CAD build for the part. Positions are in the model's coordinates, mm. Face numbers are marked on the shaded views. A direction names the side the tool comes from. Give positions to 0.01 mm unless a question says otherwise; leave off trailing zeros. Order: outer loops, then holes, each group sorted by start corner. A loop starts at its lowest first (then second) coordinate and runs counter-clockwise, first axis right, second up. Notation, with made-up numbers: M 83.5,34 L 133.5,34 A18 cw 133.5,61 Z; hole C 83.25,5 d5. An arc over 180 degrees is marked long. Put each result on its own line as item: value. Start each with the question number.
1) Cut at B-B (x = -103). Write the cut outline in (y, z).
2) Drill centre lines: line 1 (Z direction, x = -140, y = 17); line 2 (Y direction, x = -92.5, z = 20); line 3 (Y direction, x = -94, z = 9). Where is each one in solid material? Low to high. Write a range as [from, to].
3) Cut at A-A (y = 84). Write the cut outline in (x, z), and give its area (3 significant figures).
4) Pin check, flat tips, straight feed: pin 1 (7.5 mm diameter, centred on y = 74, z = -23.5, fed in from +X); pin 2 (15 mm diameter, centred on x = -15.5, z = -4.5, fed in from -Y); pin 3 (6 mm diameter, centred on x = -125, z = 15.5, fed in from +Y). Stop position of each tip, or through.
5) Tool access for the marked faces 1, 2 and 3: list every direction of +Z, -Z, +X, -X, +Y, -Y with a clear straight run to the whole face (end or side of a thin tool).
6) Cut at C-C (y = 54). Write the cut outline in (x, z), and give its area (3 significant figures).
7) Cut at D-D (y = 110). Write the cut outline in (x, z).
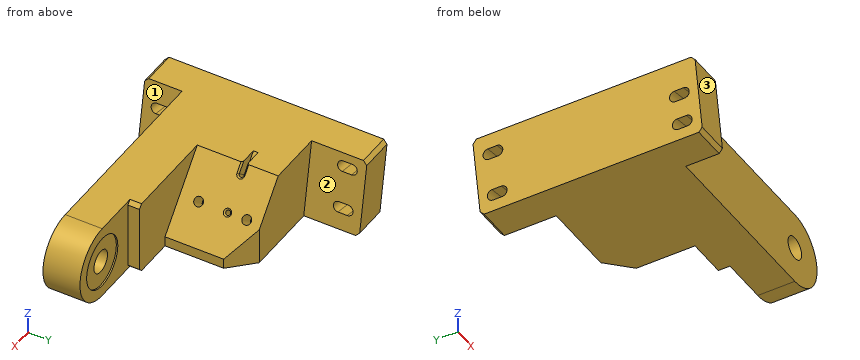
```python
from build123d import *

# Parameters (mm, degrees)
SKETCH1_W                              = 181.864
SKETCH1_H                              = 50.8
EXTRUDE1_DEPTH                         = 152.4
EXTRUDE2_DEPTH                         = 153.4
EXTRUDE3_DEPTH                         = 38.1
EXTRUDE4_DEPTH                         = 55.5498
SKETCH5_W                              = 54.61
SKETCH5_H                              = 50.8
EXTRUDE5_DEPTH                         = 7.9502
EXTRUDE6_DEPTH                         = 25.4
EXTRUDE7_DEPTH                         = 32.584173829
LPATTERN1_COUNT                        = 2
LPATTERN1_PITCH                        = 127
LPATTERN1_COUNT_DIR2                   = 2
LPATTERN1_PITCH_DIR2                   = 27.94
F_1_4_20_TAPPED_HOLE1_D                = 5.1054
F_1_4_20_TAPPED_HOLE1_DEPTH            = 16.51
F_1_4_20_TAPPED_HOLE1_CBORE_D          = 6.35
F_1_4_20_TAPPED_HOLE1_CBORE_DEPTH      = 12.7
F_1_4_20_TAPPED_HOLE1_TIP              = 1.533816902
EXTRUDE9_DEPTH                         = 128
CHAMFER1_SIZE                          = 2.54
CHAMFER2_SIZE                          = 15.24
EXTRUDE10_DEPTH                        = 32.584173829
SCREW_THRU_HOLE_AND_CBORE_D            = 15.4686
SCREW_THRU_HOLE_AND_CBORE_CBORE_D      = 35.56
SCREW_THRU_HOLE_AND_CBORE_CBORE_DEPTH  = 1.016
F_1_8_0_125_DIAMETER_HOLE1_D           = 3.19024
F_1_8_0_125_DIAMETER_HOLE1_DEPTH       = 9.525
F_1_8_0_125_DIAMETER_HOLE1_CSINK_D     = 5.334
F_1_8_0_125_DIAMETER_HOLE1_CSINK_ANGLE = 90
F_1_8_0_125_DIAMETER_HOLE1_TIP         = 0.958444791
CUT_EXTRUDE1_DEPTH                     = 9.525
CHAMFER3_SIZE                          = 1.0795


with BuildPart() as part:
    # Sketch1 → Extrude1 (new body)
    with BuildSketch(Plane(origin=(0, 0, 0), x_dir=(1, 0, 0), z_dir=(0, 1, 0))):
        with Locations((-65.532, 0)):
            Rectangle(SKETCH1_W, SKETCH1_H)
    extrude(amount=EXTRUDE1_DEPTH)

    # Sketch2 → Extrude2 (cut, through all)
    with BuildSketch(Plane(origin=(0, 152.4, 0), x_dir=(1, 0, 0), z_dir=(0, 1, 0))):
        Polygon((-156.464, -25.4), (-156.464, 25.4), (-147.50658938, 25.4), align=None)
    extrude(amount=-EXTRUDE2_DEPTH, mode=Mode.SUBTRACT)

    # Sketch3 → Extrude3 (cut)
    with BuildSketch(Plane(origin=(0, 152.4, 0), x_dir=(1, 0, 0), z_dir=(0, 1, 0))):
        Polygon((25.4, -25.4), (25.4, 25.4), (-124.39258938, 25.4), (-133.35, -25.4), align=None)
    extrude(amount=-EXTRUDE3_DEPTH, mode=Mode.SUBTRACT)

    # Sketch4 → Extrude4 (cut)
    with BuildSketch(Plane(origin=(0, 114.3, 0), x_dir=(1, 0, 0), z_dir=(0, 1, 0))):
        Polygon((25.4, -25.4), (-95.25, -25.4), (-58.42, 18.492284815), (-58.42, 25.4), (25.4, 25.4), align=None)
    extrude(amount=-EXTRUDE4_DEPTH, mode=Mode.SUBTRACT)

    # Sketch5 → Extrude5 (cut)
    with BuildSketch(Plane(origin=(0, 58.7502, 0), x_dir=(1, 0, 0), z_dir=(0, 1, 0))):
        with Locations((-1.905, 0)):
            Rectangle(SKETCH5_W, SKETCH5_H)
    extrude(amount=-EXTRUDE5_DEPTH, mode=Mode.SUBTRACT)

    # Sketch6 → Extrude6 (cut)
    with BuildSketch(Plane.XZ):
        Polygon((25.4, 25.4), (25.4, -25.4), (-124.39258938, -25.4), (-133.35, 25.4), align=None)
    extrude(amount=-EXTRUDE6_DEPTH, mode=Mode.SUBTRACT)

    # Sketch7 → Extrude7 (cut, through all)
    with BuildSketch(Plane(origin=(-124.985349671, 0, -22.03828934), x_dir=(0.173648178, 0, -0.984807753), z_dir=(0.984807753, 0, 0.173648178))):
        with BuildLine():
            Line((-35.635705397, 142.9766), (-35.635705397, 136.6266))
            ThreePointArc((-35.635705397, 136.6266), (-39.204405397, 133.0579), (-42.773105397, 136.6266))
            Line((-42.773105397, 136.6266), (-42.773105397, 142.9766))
            ThreePointArc((-42.773105397, 142.9766), (-39.204405397, 146.5453), (-35.635705397, 142.9766))
        make_face()
    extrude7 = extrude(amount=-EXTRUDE7_DEPTH, mode=Mode.SUBTRACT)

    # LPattern1: Extrude7 2 × 2, 1 skipped
    with Locations(*[Vector(0, -1, 0) * (i * LPATTERN1_PITCH) + Vector(0.173648178, 0, -0.984807753) * (j * LPATTERN1_PITCH_DIR2) for i in range(LPATTERN1_COUNT) for j in range(LPATTERN1_COUNT_DIR2) if (i, j) not in ((0, 0), (1, 0))]):
        add(extrude7, mode=Mode.SUBTRACT)

    # 1/4-20 Tapped Hole1
    with Locations(Plane(origin=(-43.387935998, 0, -36.406801094), x_dir=(0.64278761, 0, -0.766044443), z_dir=(0.766044443, 0, 0.64278761))):
        with Locations((-49.822048678, 104.648), (-49.822048678, 71.628)):
            CounterBoreHole(F_1_4_20_TAPPED_HOLE1_D / 2, F_1_4_20_TAPPED_HOLE1_CBORE_D / 2, F_1_4_20_TAPPED_HOLE1_CBORE_DEPTH, depth=F_1_4_20_TAPPED_HOLE1_DEPTH)
            with Locations((0, 0, -(F_1_4_20_TAPPED_HOLE1_DEPTH + F_1_4_20_TAPPED_HOLE1_TIP / 2))):  # 118° drill point
                Cone(0, F_1_4_20_TAPPED_HOLE1_D / 2, F_1_4_20_TAPPED_HOLE1_TIP, mode=Mode.SUBTRACT)

    # Sketch19 → Extrude9 (cut, through all)
    with BuildSketch(Plane.XZ.offset(-25.4)):
        with BuildLine():
            Line((27.94, 25.4), (0, 25.4))
            ThreePointArc((0, 25.4), (25.4, 0), (0, -25.4))
            Line((0, -25.4), (27.94, -25.4))
            Line((27.94, -25.4), (27.94, 25.4))
        make_face()
    extrude(amount=-EXTRUDE9_DEPTH, mode=Mode.SUBTRACT)

    # Chamfer1
    chamfer1_edges = [part.edges().sort_by_distance(p)[0] for p in [
        (-135.94958938, 152.4, -25.4),
        (-144.907, 0, 25.4),
        (-29.21, 54.7751, 25.4),
        (-29.21, 54.7751, -25.4),
        (-135.94958938, 0, -25.4),
        (-144.907, 152.4, 25.4),
    ]]
    chamfer(chamfer1_edges, length=CHAMFER1_SIZE)

    # Chamfer2
    chamfer2_edges = [part.edges().sort_by_distance(p)[0] for p in [
        (-58.42, 114.3, -21.946142408),
    ]]
    chamfer(chamfer2_edges, length=CHAMFER2_SIZE)

    # Sketch20 → Extrude10 (cut, through all)
    with BuildSketch(Plane(origin=(-124.985349671, 0, -22.03828934), x_dir=(0.173648178, 0, -0.984807753), z_dir=(0.984807753, 0, 0.173648178))):
        with BuildLine():
            Line((-26.745705397, 15.9766), (-26.745705397, 9.6266))
            ThreePointArc((-26.745705397, 9.6266), (-30.314405397, 6.0579), (-33.883105397, 9.6266))
            Line((-33.883105397, 9.6266), (-33.883105397, 15.9766))
            ThreePointArc((-33.883105397, 15.9766), (-30.314405397, 19.5453), (-26.745705397, 15.9766))
        make_face()
    extrude(amount=-EXTRUDE10_DEPTH, mode=Mode.SUBTRACT)

    # SCREW THRU HOLE AND CBORE (through all)
    with Locations(Plane(origin=(0, 50.8, 0), x_dir=(-1, 0, 0), z_dir=(0, 1, 0))):
        with Locations((0, 0)):
            CounterBoreHole(SCREW_THRU_HOLE_AND_CBORE_D / 2, SCREW_THRU_HOLE_AND_CBORE_CBORE_D / 2, SCREW_THRU_HOLE_AND_CBORE_CBORE_DEPTH)

    # 1/8 (0.125) Diameter Hole1
    with Locations(Plane(origin=(-43.387935998, 0, -36.406801094), x_dir=(0.64278761, 0, -0.766044443), z_dir=(0.766044443, 0, 0.64278761))):
        with Locations((-49.784, 91.412613047)):
            CounterSinkHole(F_1_8_0_125_DIAMETER_HOLE1_D / 2, F_1_8_0_125_DIAMETER_HOLE1_CSINK_D / 2, depth=F_1_8_0_125_DIAMETER_HOLE1_DEPTH, counter_sink_angle=F_1_8_0_125_DIAMETER_HOLE1_CSINK_ANGLE)
            with Locations((0, 0, -(F_1_8_0_125_DIAMETER_HOLE1_DEPTH + F_1_8_0_125_DIAMETER_HOLE1_TIP / 2))):  # 118° drill point
                Cone(0, F_1_8_0_125_DIAMETER_HOLE1_D / 2, F_1_8_0_125_DIAMETER_HOLE1_TIP, mode=Mode.SUBTRACT)

    # Sketch26 → Cut-Extrude1 (cut)
    with BuildSketch(Plane(origin=(-43.387935998, 0, -36.406801094), x_dir=(0.64278761, 0, -0.766044443), z_dir=(0.766044443, 0, 0.64278761))):
        with BuildLine():
            Line((-73.6092, 89.817493047), (-92.6592, 89.817493047))
            ThreePointArc((-92.6592, 89.817493047), (-94.25432, 91.412613047), (-92.6592, 93.007733047))
            Line((-92.6592, 93.007733047), (-73.6092, 93.007733047))
            ThreePointArc((-73.6092, 93.007733047), (-72.01408, 91.412613047), (-73.6092, 89.817493047))
        make_face()
    extrude(amount=-CUT_EXTRUDE1_DEPTH, mode=Mode.SUBTRACT)

    # Chamfer3
    chamfer3_edges = [part.edges().sort_by_distance(p)[0] for p in [
        (-92.976508859, 89.817493047, 22.690558764),
        (-92.976508859, 93.007733047, 22.690558764),
        (-89.677694345, 91.412613047, 18.759184717),
    ]]
    chamfer(chamfer3_edges, length=CHAMFER3_SIZE)


solid = part.part
```
Solution:
1. outline: M 25.4,-25.4 L 114.3,-25.4 L 114.3,25.4 L 93.01,25.4 L 93.01,19.82 L 89.82,19.82 L 89.82,25.4 L 25.4,25.4 Z
2. line 1: [-25.4, -16.72], [-9.78, 2.62], [9.57, 25.4]
2. line 2: [25.4, 89.82], [93.01, 114.3]
2. line 3: [25.4, 114.3]
3. outline: M -156.46,25.4 L -147.51,-25.4 L -58.42,-25.4 L -58.42,-18.49 L -95.25,25.4 Z
3. area: 3,940 mm²
4. pin 1: x = -58.42
4. pin 2: y = 25.4
4. pin 3: y = 114.3
5. face 1: +Z, +X, -Y
5. face 2: +Z, +X, +Y
5. face 3: +Z, -Z, +X, -X, -Y
6. outline: M -156.46,25.4 L -147.51,-25.4 L -31.75,-25.4 L -29.21,-22.86 L -29.21,22.86 L -31.75,25.4 Z
6. area: 6,230 mm²
7. outline: M -156.46,25.4 L -147.51,-25.4 L -69.36,-25.4 L -69.36,-5.45 L -95.25,25.4 Z
